from build123d import *

# Parameters (mm, degrees)
F0_R     = 95.25
F2_DEPTH = 3.175
F1_R     = 22.86
F3_DEPTH = 25.4
F5_DEPTH = 25.4


with BuildPart() as f2:
    # F0 (on Front) → F2 (new body)
    with BuildSketch(Plane.XZ):
        Circle(F0_R)
    extrude(amount=F2_DEPTH)

    # F1 (on face) → F3 (cut)
    with BuildSketch(Plane.XZ):
        Circle(F1_R)
    extrude(amount=F3_DEPTH, mode=Mode.SUBTRACT)

    # F4 (on face) → F5 (cut)
    with BuildSketch(Plane.XZ.offset(3.175)):
        Polygon((-81.28, -8.980256), (-72.299744, 0), (-81.28, 8.980256), (-90.260256, 0), align=None)
        Polygon((0, -90.260256), (8.980256, -81.28), (0, -72.299744), (-8.980256, -81.28), align=None)
        Polygon((90.260256, 0), (81.28, 8.980256), (72.299744, 0), (81.28, -8.980256), align=None)
        Polygon((0, 90.260256), (-8.980256, 81.28), (0, 72.299744), (8.980256, 81.28), align=None)
    extrude(amount=-F5_DEPTH, mode=Mode.SUBTRACT)


solid = f2.part
Input: part model. Units: mm. Frame: model coordinates. Coordinates: 2 decimals unless noted, no trailing zeros. Loops run counter-clockwise (first coordinate to the right, second up) from the corner with the lowest first, then second, coordinate; pieces in that order, holes last. Notation, with made-up numbers: (53, -3.5) -> (73, -3.5) arc R20 cw to (73, 7.5) -> close; hole circle Ø8 at (-33.75, -39.75). An arc over 180 degrees is marked (long way). One line per item, written item: value.
(1) Cut plane C-C (z = 12). Output: boundary loops of the cut face in (x, y) (3 decimals), then the cut area to 3 significant figures.
Answer below:
outline: (-94.491, -3.175) -> (-19.457, -3.175) -> (-19.457, 0) -> (-94.491, 0) -> close; (19.457, -3.175) -> (94.491, -3.175) -> (94.491, 0) -> (19.457, 0) -> close
area: 476 mm2
(2) Pin query (flat end, axial travel): pin 1 Ø1 at (y, z) = (-2.5, -59) entering from +X; pin 2 Ø1 at (x, y) = (54, -0.5) entering from -Z; pin 3 Ø1.5 at (y, z) = (-3, 24.5) entering from -X. Return the tip coordinate at first contact, or that it passes through.
Answer below:
pin 1: stops at x = 75.17
pin 2: stops at z = -78.81
pin 3: stops at x = -92.24
(3) Cut plane A-A (y = -2.45). Output: boundary loops of the cut face in (x, z).
Answer below:
outline: circle Ø190.5 at (0, 0); hole (-90.26, 0) -> (-81.28, -8.98) -> (-72.3, 0) -> (-81.28, 8.98) -> close; hole circle Ø45.72 at (0, 0); hole (-8.98, -81.28) -> (0, -90.26) -> (8.98, -81.28) -> (0, -72.3) -> close; hole (-8.98, 81.28) -> (0, 72.3) -> (8.98, 81.28) -> (0, 90.26) -> close; hole (72.3, 0) -> (81.28, -8.98) -> (90.26, 0) -> (81.28, 8.98) -> close
(4) Cut plane B-B (x = -20). Output: boundary loops of the cut face in (y, z) (3 decimals), then the cut area to 3 significant figures.
Answer below:
outline: (-3.175, -93.127) -> (0, -93.127) -> (0, -11.072) -> (-3.175, -11.072) -> close; (-3.175, 11.072) -> (0, 11.072) -> (0, 93.127) -> (-3.175, 93.127) -> close
area: 521 mm2
(5) Draft query along Z for faces 1 (the face through (-75.587, -1.565, -57.958)), 2 (the face through (-4.43, -1.61, 85.83)), 3 (the face through (20, -3.175, -20)). Return one class per face: pulls with the +Z half, pulls with the -Z half, needs draft (parallel to the pull), parting line crosses it, or undercut.
Answer below:
face 1: parting line crosses it
face 2: undercut
face 3: needs draft
(6) Cut plane D-D (z = -66). Output: boundary loops of the cut face in (x, y) (3 decimals), then the cut area to 3 significant figures.
Answer below:
outline: (-68.677, -3.175) -> (68.677, -3.175) -> (68.677, 0) -> (-68.677, 0) -> close
area: 436 mm2
(7) Ray query, line 1 along Z through (x, y) = (0, -1.75); line 2 along Z through (x, y) = (-0.5, -0.45); line 3 along X through (y, z) = (-2.65, -2.5). Return the intervals inside material, ascending.
Answer below:
line 1: z = -95.25 to -90.26, -72.3 to -22.86, 22.86 to 72.3, 90.26 to 95.25
line 2: z = -95.25 to -89.76, -72.8 to -22.85, 22.85 to 72.8, 89.76 to 95.25
line 3: x = -95.22 to -87.76, -74.8 to -22.72, 22.72 to 74.8, 87.76 to 95.22
